Geometry: final body of the model. Coordinates: model frame, mm. A direction names the side the tool comes from. Round coordinates to 2 decimals unless told otherwise and drop trailing zeros. Loops run counter-clockwise (first coordinate to the right, second up) from the corner with the lowest first, then second, coordinate; pieces in that order, holes last. Notation, with made-up numbers: (41.25, 49.5) -> (62.25, 49.5) arc R21 cw to (62.25, 80.5) -> close; hole circle Ø9 at (86.5, 20.25). An arc over 180 degrees is marked (long way). Answer in a Markdown table with one row per item.
```python
from build123d import *

# Parameters (mm, degrees)
F0_W     = 762
F0_H     = 711.2
F0_W_2   = 660.4
F0_H_2   = 609.6
F1_DEPTH = 25.4
F3_DEPTH = 25.4


with BuildPart() as f1:
    # F0 (on Front) → F1 (new body, symmetric)
    with BuildSketch(Plane.XZ):
        Rectangle(F0_W, F0_H)
        Rectangle(F0_W_2, F0_H_2, mode=Mode.SUBTRACT)
    extrude(amount=F1_DEPTH, both=True)

    # F2 (on Front) → F3 (join, symmetric)
    with BuildSketch(Plane.XZ):
        Polygon((-381, 25.4), (-381, 0), (-381, -25.4), (381, -25.4), (381, 0), (381, 25.4), align=None)
    extrude(amount=F3_DEPTH, both=True)


solid = f1.part
```
Item 1: Draft query along X for faces 3 (the face through (-330.2, 0, 163)), 4 (the face through (-5, 0, -355.6)), 5 (the face through (-381, 0, 5)). Return one class per face: pulls with the +X half, pulls with the -X half, needs draft (parallel to the pull), parting line crosses it, or undercut.
Answer:
| item | result |
|---|---|
| face 3 | undercut |
| face 4 | needs draft |
| face 5 | pulls with the -X half |
Item 2: Reachability of faces 1 (the face through (-330.2, 0, -167)), 2 (the face through (381, 0, -5)) from +Z, -Z, +X, -X, +Y, -Y: full face, straight path, thin tool, end or side. Return the list, or none.
Answer:
| item | result |
|---|---|
| face 1 | +Y, -Y |
| face 2 | +Z, -Z, +X, +Y, -Y |
Item 3: Cut plane B-B (x = -8). Output: boundary loops of the cut face in (y, z).
Answer:
| item | result |
|---|---|
| outline | (-25.4, -355.6) -> (25.4, -355.6) -> (25.4, -304.8) -> (-25.4, -304.8) -> close; (-25.4, -25.4) -> (25.4, -25.4) -> (25.4, 25.4) -> (-25.4, 25.4) -> close; (-25.4, 304.8) -> (25.4, 304.8) -> (25.4, 355.6) -> (-25.4, 355.6) -> close |
Item 4: Cut plane A-A (z = -53). Output: boundary loops of the cut face in (x, y), then the cut area to 3 significant figures.
Answer:
| item | result |
|---|---|
| outline | (-381, -25.4) -> (-330.2, -25.4) -> (-330.2, 25.4) -> (-381, 25.4) -> close; (330.2, -25.4) -> (381, -25.4) -> (381, 25.4) -> (330.2, 25.4) -> close |
| area | 5,160 mm² |
Item 5: Cut plane C-C (y = 7). Output: boundary loops of the cut face in (x, z), then the cut area to 3 significant figures.
Answer:
| item | result |
|---|---|
| outline | (-381, -355.6) -> (381, -355.6) -> (381, 355.6) -> (-381, 355.6) -> close; hole (-330.2, -304.8) -> (330.2, -304.8) -> (330.2, -25.4) -> (-330.2, -25.4) -> close; hole (-330.2, 25.4) -> (330.2, 25.4) -> (330.2, 304.8) -> (-330.2, 304.8) -> close |
| area | 173,000 mm² |
Item 6: Line query: probe 1 along Z at (x, y) = (100, 21.5); probe 2 along X at (y, z) = (16.5, -89). Output: solid intervals per line, ascending. Write a range as [from, to].
Answer:
| item | result |
|---|---|
| probe 1 | z = [-355.6, -304.8], [-25.4, 25.4], [304.8, 355.6] |
| probe 2 | x = [-381, -330.2], [330.2, 381] |
